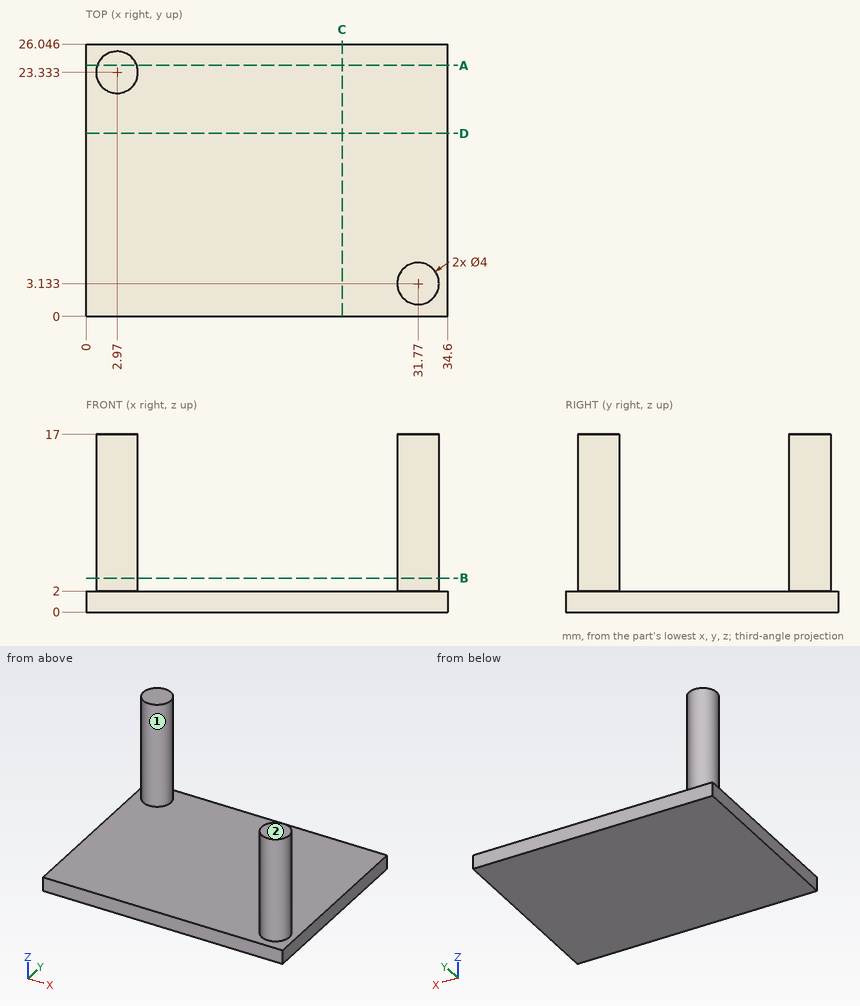
The drawing under review shows one solid part. Ordinate dimensions are in mm from its lowest x, y, z. A direction names the side the tool comes from. Give positions to 0.01 mm unless a question says otherwise; leave off trailing zeros. Order: outer loops, then holes, each group sorted by start corner. A loop starts at its lowest first (then second) coordinate and runs counter-clockwise, first axis right, second up. Notation, with made-up numbers: (-21, -25) -> (-12, -25) arc R29 cw to (-12, 10) -> close; hole circle Ø9 at (-11, 54.25). An arc over 180 degrees is marked (long way). Write item = value, one per line. Start each with the question number.
(1) We need section A-A on y = 24. Write out the cut boundary in (x, z) (1 decimal), plus the area to 3 significant figures.
(2) We need section C-C on x = 24.5. Write out the cut boundary in (y, z).
(3) We need section D-D on y = 17.5. Write out the cut boundary in (x, z).
(4) For pin 1 (8 mm diameter, centred on x = 21, y = 12, fed in from +Z), flat-tipped, find the tip position at first contact; note if it passes through.
(5) For the marked faces 1 and 2, list the 3-axis set-ups (+Z, -Z, +X, -X, +Y, -Y) from which the entire face can be reached by the end or side of a thin tool; tool diameter is ignored.
(6) We need section B-B on z = 3.25. Write out the cut boundary in (x, y).
(7) To check wall thickness, follow line 1 along Z through (x, y) = (14.5, 13.25); line 2 along X through (y, z) = (3, 6.5) (1 decimal); line 3 along Y through (x, z) = (30.5, 15.25). State the ranges of each line that lie inside material, in increasing order.
Numbers:
q1.outline = (0, 0) -> (34.6, 0) -> (34.6, 2) -> (4.9, 2) -> (4.9, 17) -> (1.1, 17) -> (1.1, 2) -> (0, 2) -> close
q1.area = 126 mm^2
q2.outline = (0, 0) -> (26.05, 0) -> (26.05, 2) -> (0, 2) -> close
q3.outline = (0, 0) -> (34.6, 0) -> (34.6, 2) -> (0, 2) -> close
q4.pin_1 = 2
q5.face_1 = +Z
q5.face_2 = +Z, +X, -X, +Y, -Y
q6.outline = circle Ø4 at (2.97, 23.33); circle Ø4 at (31.77, 3.13)
q7.line_1 = 0 to 2
q7.line_2 = 29.8 to 33.8
q7.line_3 = 1.59 to 4.68
